Model file for the job. Use its own axes, mm. Face numbers are marked on the shaded views. A direction names the side the tool comes from. Round coordinates to 2 decimals unless told otherwise and drop trailing zeros. Use a Markdown table: item, result. Add a question column.
Item 1: Two-plate mould, pull along X, no slides. Class the marked faces 3, 4, 5 and 6: +X half, -X half, draft (parallel to the pull), parting line (faces both ways), or undercut.
Item 2: Saw through at A-A on z = -18. Give the number of separate pieces and of enclosed holes in the cut face, then the cut area to 3 significant figures.
Item 3: Pin check, flat tips, straight feed: P1, Ø16, axis at x = -20, y = -17, coming from the +Z side; P2, Ø1.5, axis at x = 31, z = -63.5, coming from the +Y side; P3, Ø25, axis at x = -5, z = -25.5, coming from the -Y side; P4, Ø5, axis at y = -21, z = -45.5, coming from the -X side. Stop position of each tip, or through.
Item 4: Tool access for the marked faces 1 and 2: list every direction of +Z, -Z, +X, -X, +Y, -Y with a clear straight run to the whole face (end or side of a thin tool).
Item 5: Wall check: L1, parallel to X at y = 27, z = -47; L2, parallel to Y at x = -20, z = -65; L3, parallel to X at y = 5, z = -32. Give the ranges that are in metal, low to high. Write a range as from..to.
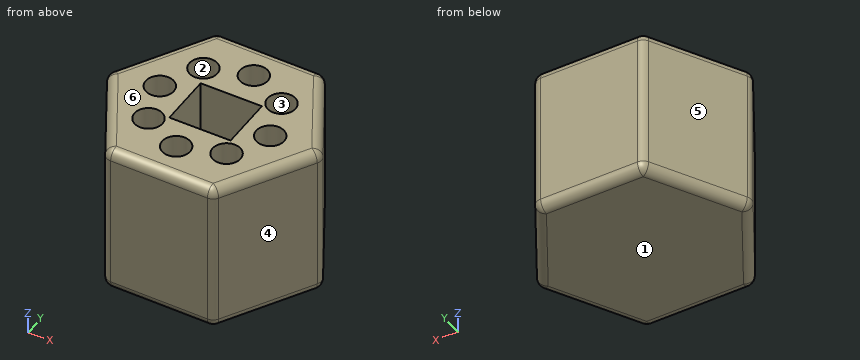
```python
from build123d import *

# Parameters (mm, degrees)
F1_DEPTH = 80
F2_R     = 5
F3_R     = 7.212023
F4_DEPTH = 50
F5_DEPTH = 70
F6_W     = 31.557379
F6_H     = 27.543242
F7_DEPTH = 50


with BuildPart() as f1:
    # F0 (on Top) → F1 (new body)
    with BuildSketch(Plane.XY):
        Polygon((27.461036, -48.6942), (55.900933, -0.565146), (28.439897, 48.129055), (-27.461036, 48.6942), (-55.900933, 0.565146), (-28.439897, -48.129055), align=None)
    extrude(amount=-F1_DEPTH)

    # F2
    f2_edges = [f1.edges().sort_by_distance(p)[0] for p in [
        (55.900933, -0.565146, -40),
        (27.461036, -48.6942, -40),
        (41.680984, -24.629673, -80),
        (41.680984, -24.629673, 0),
        (-0.48943, -48.411628, 0),
        (-0.48943, -48.411628, -80),
        (-28.439897, -48.129055, -40),
        (42.170415, 23.781955, -80),
        (42.170415, 23.781955, 0),
        (28.439897, 48.129055, -40),
        (0.48943, 48.411628, 0),
        (-41.680984, 24.629673, 0),
        (-42.170415, -23.781955, 0),
        (0.48943, 48.411628, -80),
        (-41.680984, 24.629673, -80),
        (-42.170415, -23.781955, -80),
        (-55.900933, 0.565146, -40),
        (-27.461036, 48.6942, -40),
    ]]
    fillet(f2_edges, radius=F2_R)

    # F3 (on face) → F4 (join)
    with BuildSketch(Plane.XY):
        with Locations((-19.36131, 22.915926)):
            Circle(F3_R)
        with Locations((-29.89452, 2.513494)):
            Circle(F3_R)
        with Locations((-22.915926, -19.36131)):
            Circle(F3_R)
        with Locations((-2.513494, -29.89452)):
            Circle(F3_R)
        with Locations((19.36131, -22.915926)):
            Circle(F3_R)
        with Locations((29.89452, -2.513494)):
            Circle(F3_R)
        with Locations((22.915926, 19.36131)):
            Circle(F3_R)
        with Locations((2.513494, 29.89452)):
            Circle(F3_R)
    extrude(amount=-F4_DEPTH)

    # F3 (on face) → F5 (cut)
    with BuildSketch(Plane.XY):
        with Locations((-29.89452, 2.513494)):
            Circle(F3_R)
        with Locations((-22.915926, -19.36131)):
            Circle(F3_R)
        with Locations((19.36131, -22.915926)):
            Circle(F3_R)
        with Locations((2.513494, 29.89452)):
            Circle(F3_R)
        with Locations((-2.513494, -29.89452)):
            Circle(F3_R)
        with Locations((-19.36131, 22.915926)):
            Circle(F3_R)
        with Locations((22.915926, 19.36131)):
            Circle(F3_R)
        with Locations((29.89452, -2.513494)):
            Circle(F3_R)
    extrude(amount=-F5_DEPTH, mode=Mode.SUBTRACT)

    # F6 (on face) → F7 (cut)
    with BuildSketch(Plane.XY):
        with Locations((0.573771, -0.422957)):
            Rectangle(F6_W, F6_H)
    extrude(amount=-F7_DEPTH, mode=Mode.SUBTRACT)


solid = f1.part
```
Entries:
| question | item | result |
|---|---|---|
| 1 | face 3 | undercut |
| 1 | face 4 | +X half |
| 1 | face 5 | -X half |
| 1 | face 6 | draft |
| 2 | separate pieces | 1 |
| 2 | enclosed holes | 9 |
| 2 | area | 5,940 mm2 |
| 3 | P1 | z = 0 |
| 3 | P2 | y = 44.92 |
| 3 | P3 | y = -48.49 |
| 3 | P4 | x = -45.15 |
| 4 | face 1 | -Z, +X, -X, +Y, -Y |
| 4 | face 2 | +Z |
| 5 | L1 | -40.28..-25.31, -13.42..-4.09, 9.12..40.36 |
| 5 | L2 | -48.21..-25.96, -12.77..15.73, 30.1..48.62 |
| 5 | L3 | -53.28..-36.66, -23.12..-15.2, 16.35..52.76 |
